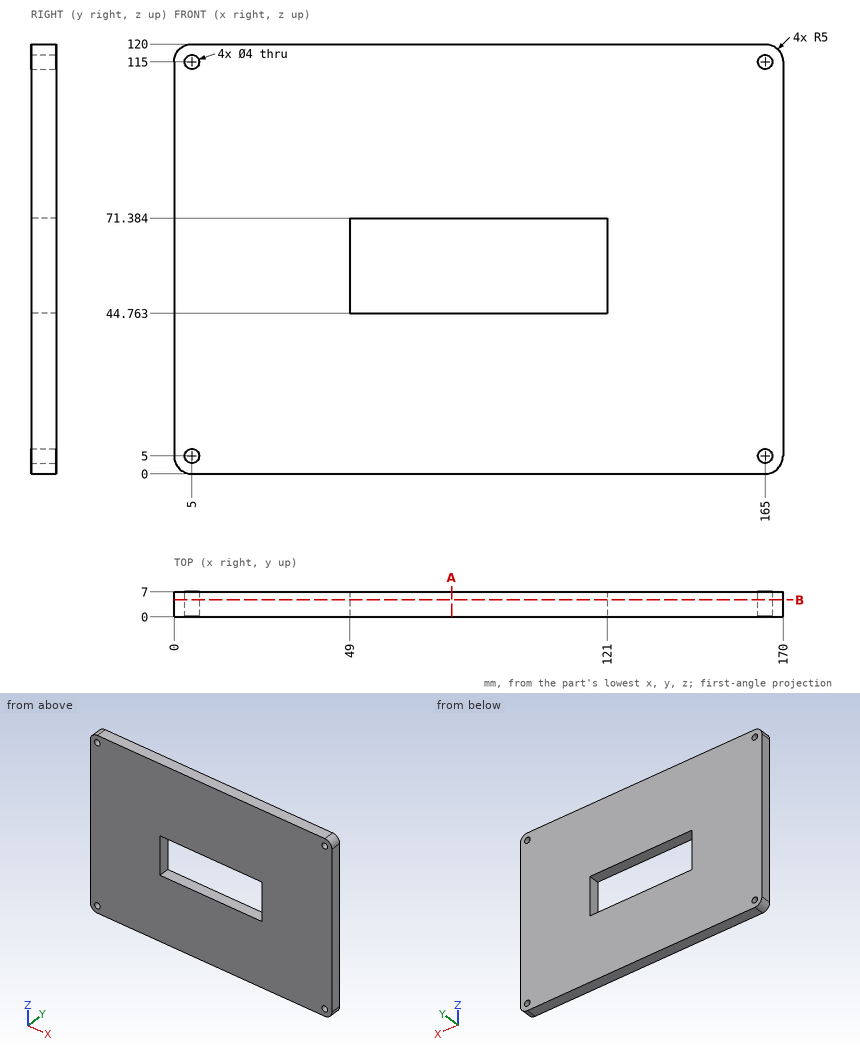
Can you work these out from the drawing? Everything is in mm from the part's minimum corner. Round coordinates to 2 decimals unless told otherwise and drop trailing zeros. Write each loop counter-clockwise with the first axis right and the second up, starting at its lowest first coordinate (ties: lowest second). Pieces come first, ordered by that corner, then holes. Notation, with made-up numbers: M -36,-25 L -13,-25 A17 ccw -13,-8 Z; hole C -11.75,86 d4. An arc over 180 degrees is marked long. Use a Markdown table: item, result.
Item 1: I want a section at B-B (y = 4.75). List the corners of the cut face in (x, z) for me.
Found:
| item | result |
|---|---|
| outline | M 0,5 A5 ccw 5,0 L 165,0 A5 ccw 170,5 L 170,115 A5 ccw 165,120 L 5,120 A5 ccw 0,115 Z; hole C 5,5 d4; hole C 5,115 d4; hole M 49,44.76 L 121,44.76 L 121,71.38 L 49,71.38 Z; hole C 165,5 d4; hole C 165,115 d4 |
Item 2: I want a section at A-A (x = 77.5). List the corners of the cut face in (y, z) for me, and give its area (3 significant figures).
Found:
| item | result |
|---|---|
| outline | M 0,0 L 7,0 L 7,44.76 L 0,44.76 Z; M 0,71.38 L 7,71.38 L 7,120 L 0,120 Z |
| area | 654 mm2 |
Item 3: If I drill on line 1 along Z through (x, y) = (5, 1.5); line 2 along X through (y, z) = (2.75, 5); line 3 along Z through (x, y) = (88, 0.5), over which ranges is the centre line in solid material (lowest first)? Write a range as [from, to].
Found:
| item | result |
|---|---|
| line 1 | z = [0, 3], [7, 113], [117, 120] |
| line 2 | x = [0, 3], [7, 163], [167, 170] |
| line 3 | z = [0, 44.76], [71.38, 120] |
